```python
from build123d import *

# Parameters (mm, degrees)
F9_W       = 40
F9_H       = 60
F0_DEPTH   = 47.5
F10_W      = 81.115219
F10_H      = 40
F1_DEPTH   = 37.5
F3_R       = 12.5
F3_R_2     = 7.5
F4_DEPTH   = 5
F2_R       = 12.5
F2_R_2     = 7.5
F11_DEPTH  = 5
F5_R       = 10
F12_R      = 15
F12_R_2    = 10
F13_DEPTH  = 5
F6_DEPTH   = 25
F4_FACE_R  = 7.5
F7_DEPTH   = 25
F13_FACE_R = 10
F8_DEPTH   = 25


with BuildPart() as f0:
    # F9 (on Front) → F0 (new body)
    with BuildSketch(Plane.XZ):
        Rectangle(F9_W, F9_H)
    extrude(amount=F0_DEPTH)

    # F10 (on Front) → F1 (cut)
    with BuildSketch(Plane.XZ):
        with Locations((-0.543405, 0)):
            Rectangle(F10_W, F10_H)
    extrude(amount=F1_DEPTH, mode=Mode.SUBTRACT)

    # F3 (on face) → F4 (join)
    with BuildSketch(Plane(origin=(0, 0, -30), x_dir=(1, 0, 0), z_dir=(0, 0, -1))):
        with Locations((0, 20)):
            Circle(F3_R)
        with Locations((0, 20)):
            Circle(F3_R_2, mode=Mode.SUBTRACT)
    extrude(amount=F4_DEPTH)

    # F2 (on face) → F11 (join)
    with BuildSketch(Plane.XY.offset(30)):
        with Locations((0, -20)):
            Circle(F2_R)
        with Locations((0, -20)):
            Circle(F2_R_2, mode=Mode.SUBTRACT)
    extrude(amount=F11_DEPTH)

    # F5
    f5_edges = [f0.edges().sort_by_distance(p)[0] for p in [
        (0, -47.5, -30),
        (0, -47.5, 30),
        (20, 0, -25),
        (20, 0, 25),
        (-20, 0, 25),
        (-20, 0, -25),
    ]]
    fillet(f5_edges, radius=F5_R)

    # F12 (on face) → F13 (join)
    with BuildSketch(Plane.XZ.offset(47.5)):
        Circle(F12_R)
        Circle(F12_R_2, mode=Mode.SUBTRACT)
    extrude(amount=F13_DEPTH)

    # F2 (on face) → F6 (cut)
    with BuildSketch(Plane.XY.offset(30)):
        with Locations((0, -20)):
            Circle(F2_R_2)
    extrude(amount=-F6_DEPTH, mode=Mode.SUBTRACT)

    # F4_face (on face) → F7 (cut)
    with BuildSketch(Plane(origin=(0, -20, -30), x_dir=(1, 0, 0), z_dir=(0, 0, -1))):
        Circle(F4_FACE_R)
    extrude(amount=-F7_DEPTH, mode=Mode.SUBTRACT)

    # F13_face (on face) → F8 (cut)
    with BuildSketch(Plane.XZ.offset(47.5)):
        Circle(F13_FACE_R)
    extrude(amount=-F8_DEPTH, mode=Mode.SUBTRACT)


solid = f0.part
```
CAD build for the part. Positions are in the model's coordinates, mm. A direction names the side the tool comes from. Coordinates: 2 decimals unless noted, no trailing zeros. Write each loop counter-clockwise with the first axis right and the second up, starting at its lowest first coordinate (ties: lowest second). Pieces come first, ordered by that corner, then holes.
(1) Cut at C-C, the plane z = 0. List the corners of the cut face in (x, y), and give its area (3 significant figures).
(2) 3-axis set-ups, long thin cutter, end or side, ignore diameter. For faces 1 (the face through (9, -10, -30)), 2 (the face through (9, -47.5, 14)), 3 (the face through (0, -10, -20)), 4 (the face through (-2.71, -32.203, 32.465)): which of +Z, -Z, +X, -X, +Y, -Y reach the whole face in a straight line?
(3) Cut at A-A, the plane y = -20. List the corners of the cut face in (x, z).
(4) Cut at D-D, the plane x = 16. List the corners of the cut face in (y, z), and give its area (3 significant figures).
(5) Drill centre lines: probe 1 along Z at (x, y) = (17.5, -23.5); probe 2 along X at (y, z) = (-20, -32); probe 3 along Y at (x, z) = (0, -33). Where is each one in solid material? Low to high.
(6) Flat gauge pins, fed straight in: pin 1 (8 mm diameter, centred on x = 15.5, y = -6, fed in from +Z); pin 2 (9 mm diameter, centred on x = 0, y = -20, fed in from +Z); pin 3 (11 mm diameter, centred on x = 3.5, y = -26, fed in from -Z); pin 4 (4 mm diameter, centred on x = 11, y = -45.5, fed in from -Z). Where does each tip first touch, or does it go through?
(7) Cut at B-B, the plane x = 0. Count the separate pieces of the cut face and the enclosed holes in it, and give its area (3 significant figures).
Geometry says:
1. outline: (-20, -47.5) - (-15, -47.5) - (-15, -52.5) - (-10, -52.5) - (-10, -37.5) - (-20, -37.5) - close; (10, -52.5) - (15, -52.5) - (15, -47.5) - (20, -47.5) - (20, -37.5) - (10, -37.5) - close
1. area: 250 mm2
2. face 1: -Z
2. face 2: -Y
2. face 3: +X, -X, +Y
2. face 4: +Z
3. outline: (-20, -30) - (-12.5, -30) - (-12.5, -35) - (-7.5, -35) - (-7.5, -20) - (-20, -20) - close; (-20, 20) - (-7.5, 20) - (-7.5, 35) - (-12.5, 35) - (-12.5, 30) - (-20, 30) - close; (7.5, -35) - (12.5, -35) - (12.5, -30) - (20, -30) - (20, -20) - (7.5, -20) - close; (7.5, 20) - (20, 20) - (20, 30) - (12.5, 30) - (12.5, 35) - (7.5, 35) - close
4. outline: (-47.5, -20) arc R10 ccw to (-37.5, -30) - (-2, -30) - (-2, -20) - (-37.5, -20) - (-37.5, 20) - (-2, 20) - (-2, 30) - (-37.5, 30) arc R10 ccw to (-47.5, 20) - close
4. area: 1,270 mm2
5. probe 1: z = -30 to -20, 20 to 30
5. probe 2: x = -12.5 to -7.5, 7.5 to 12.5
5. probe 3: y = -32.5 to -27.5, -12.5 to -7.5
6. pin 1: stops at z = 30
6. pin 2: passes through
6. pin 3: stops at z = -35
6. pin 4: stops at z = -28
7. separate pieces: 4
7. enclosed holes: 0
7. area: 957 mm2
